Can you work these out from the model? Positions are in its coordinate system, mm. A direction names the side the tool comes from. Round coordinates to 2 decimals unless told otherwise and drop trailing zeros. Order: outer loops, then holes, each group sorted by start corner. A loop starts at its lowest first (then second) coordinate and runs counter-clockwise, first axis right, second up. Notation, with made-up numbers: (39, 9.25) -> (64, 9.25) arc R22 cw to (64, 29.25) -> close; hole circle Ø7 at (7.25, 55). An arc over 180 degrees is marked (long way). Use a Markdown table: item, result. Add a question column.
Q1. For faces 4 (the face through (12, 28, 35)), 5 (the face through (35.651, -4.868, 22.325)), 6 (the face through (-0.66, -29.993, 117.902)), 7 (the face through (-31, 0, 95)), which set-ups out of +Z, -Z, +X, -X, +Y, -Y let a thin tool reach every point of the face, with its end or its side?
Q2. I need wall thicknesses on line 1 along Y through (x, z) = (0, 18); line 2 along Z through (x, y) = (-42.5, -6.5); line 3 along Y through (x, z) = (0, 6.5). Which ranges of each line are inside material? Lowest first, please. Write a range as [from, to].
Q3. If we section it at D-D on z = 57: List the corners of the cut face in (x, y) for me.
Q4. We'd pull the mould along X, two halves only. Please class faces 1 (the face through (-59.94, 2.64, 17.26)), 2 (the face through (31, -18, 76)), 3 (the face through (-48.4, -15.2, 88.1)): +X half, -X half, draft (parallel to the pull), parting line (faces both ways), or undercut.
Q5. If we section it at A-A on z = 88: List the corners of the cut face in (x, y) for me.
Q6. I'm going to push flat-ended pins straight in: pin 1 Ø4 at (x, z) = (-26.5, 100.5) entering from -Y; pin 2 Ø10 at (x, z) = (-46, 26.5) entering from -Y; pin 3 Ø14.5 at (x, y) = (-42, 0) entering from -Z. Where does each tip first touch, or does it pass through?
Q7. If we section it at C-C on x = -45: List the corners of the cut face in (y, z) for me.
Q8. If we section it at B-B on y = -38.5: List the corners of the cut face in (x, z) for me, plus the area to 3 significant figures.
```python
from build123d import *

# Parameters (mm, degrees)
BOSS_EXTRUDE1_DEPTH         = 125
SKETCH1_4_R                 = 12.5
BOSS_EXTRUDE2_DEPTH         = 65
SKETCH1_5_R                 = 60
SKETCH1_5_R_2               = 8
SKETCH1_5_R_3               = 30
BOSS_EXTRUDE3_DEPTH         = 35
BOSS_EXTRUDE4_START         = -49
BOSS_EXTRUDE4_DEPTH         = 35
FILLET1_RADIUS              = 17.5
FILLET1_LENGTH              = 30
F_16_0_16_DIAMETER_HOLE1_D  = 16
FILLET1_OF_MIRROR1_2_RADIUS = 17.5
FILLET1_OF_MIRROR1_2_LENGTH = 30
SKETCH5_R                   = 53.79037733
CUT_EXTRUDE2_DEPTH          = 10


with BuildPart() as part:
    # Sketch1 → Boss-Extrude1 (new body)
    with BuildSketch(Plane.XY):
        with BuildLine():
            Line((30, 0), (20, 0))
            ThreePointArc((20, 0), (0, -20), (-20, 0))
            Line((-20, 0), (-30, 0))
            ThreePointArc((-30, 0), (0, -30), (30, 0))
        make_face()
    extrude(amount=BOSS_EXTRUDE1_DEPTH)

    # Sketch1<4> → Boss-Extrude2 (add)
    with BuildSketch(Plane.XY):
        with BuildLine():
            ThreePointArc((-20, 0), (0, -20), (20, 0))
            Line((20, 0), (30, 0))
            ThreePointArc((30, 0), (0, 30), (-30, 0))
            Line((-30, 0), (-20, 0))
        make_face()
        Circle(SKETCH1_4_R, mode=Mode.SUBTRACT)
    extrude(amount=BOSS_EXTRUDE2_DEPTH)

    # Sketch1<5> → Boss-Extrude3 (add)
    with BuildSketch(Plane.XY):
        Circle(SKETCH1_5_R)
        with Locations((0, 42)):
            Circle(SKETCH1_5_R_2, mode=Mode.SUBTRACT)
        with Locations((-42, 0)):
            Circle(SKETCH1_5_R_2, mode=Mode.SUBTRACT)
        with Locations((0, -42)):
            Circle(SKETCH1_5_R_2, mode=Mode.SUBTRACT)
        with Locations((42, 0)):
            Circle(SKETCH1_5_R_2, mode=Mode.SUBTRACT)
        Circle(SKETCH1_5_R_3, mode=Mode.SUBTRACT)
    extrude(amount=BOSS_EXTRUDE3_DEPTH)

    # Sketch2 → Boss-Extrude4 (add)
    with BuildSketch(Plane.XY.offset(125).offset(BOSS_EXTRUDE4_START)):
        with BuildLine():
            Line((30, 0), (60, 0))
            Line((60, 0), (60, -26.364821455))
            Line((60, -26.364821455), (60, -30))
            Line((60, -30), (0, -30))
            ThreePointArc((0, -30), (21.213203436, -21.213203436), (30, 0))
        make_face()
    boss_extrude4 = extrude(amount=BOSS_EXTRUDE4_DEPTH)

    # Fillet1: full round fillet: the end face becomes a half cylinder, R = half its width
    fillet1_face = Plane((60, -15, 93.5), x_dir=(0, 1, 0), z_dir=(1, 0, 0))  # on the end face: x along it, z out of the body
    fillet1_slab = fillet1_face.offset(-FILLET1_RADIUS / 2) * Box(FILLET1_LENGTH, 2 * FILLET1_RADIUS, FILLET1_RADIUS, mode=Mode.PRIVATE)  # the body's end, R deep
    fillet1_round = Plane((42.5, -15, 93.5), x_dir=(1, 0, 0), z_dir=(0, 1, 0)) * Cylinder(FILLET1_RADIUS, FILLET1_LENGTH, mode=Mode.PRIVATE)  # its axis R under the face
    add(fillet1_slab - fillet1_round, mode=Mode.SUBTRACT)

    # Ø16.0 (16) Diameter Hole1 (through all)
    with Locations(Plane(origin=(42.5, 0, 93.5), x_dir=(1, 0, 0), z_dir=(0, 1, 0))):
        with Locations((0, 0)):
            f_16_0_16_diameter_hole1 = Hole(F_16_0_16_DIAMETER_HOLE1_D / 2)

    # Mirror1: Boss-Extrude4, Ø16.0 (16) Diameter Hole1 across plane
    add(boss_extrude4.mirror(Plane(origin=(0, 0, 0), x_dir=(0, 0, 1), z_dir=(1, 0, 0))))
    add(f_16_0_16_diameter_hole1.mirror(Plane(origin=(0, 0, 0), x_dir=(0, 0, 1), z_dir=(1, 0, 0))), mode=Mode.SUBTRACT)

    # Fillet1 of Mirror1 2: full round fillet: the end face becomes a half cylinder, R = half its width
    fillet1_of_mirror1_2_face = Plane((-60, -15, 93.5), x_dir=(0, 1, 0), z_dir=(-1, 0, 0))  # on the end face: x along it, z out of the body
    fillet1_of_mirror1_2_slab = fillet1_of_mirror1_2_face.offset(-FILLET1_OF_MIRROR1_2_RADIUS / 2) * Box(FILLET1_OF_MIRROR1_2_LENGTH, 2 * FILLET1_OF_MIRROR1_2_RADIUS, FILLET1_OF_MIRROR1_2_RADIUS, mode=Mode.PRIVATE)  # the body's end, R deep
    fillet1_of_mirror1_2_round = Plane((-42.5, -15, 93.5), x_dir=(-1, 0, 0), z_dir=(0, 1, 0)) * Cylinder(FILLET1_OF_MIRROR1_2_RADIUS, FILLET1_OF_MIRROR1_2_LENGTH, mode=Mode.PRIVATE)  # its axis R under the face
    add(fillet1_of_mirror1_2_slab - fillet1_of_mirror1_2_round, mode=Mode.SUBTRACT)

    # Sketch5 → Cut-Extrude2 (cut)
    with BuildSketch(Plane(origin=(0, 0, 0), x_dir=(-1, 0, 0), z_dir=(0, 0, -1))):
        Circle(SKETCH5_R)
    extrude(amount=-CUT_EXTRUDE2_DEPTH, mode=Mode.SUBTRACT)


solid = part.part
```
Answer below:
| question | item | result |
|---|---|---|
| 1 | face 4 | none |
| 1 | face 5 | -Z |
| 1 | face 6 | +Z, -Y |
| 1 | face 7 | +Z, +X, -X, +Y |
| 2 | line 1 | [-60, -50], [-34, -12.5], [12.5, 34], [50, 60] |
| 2 | line 2 | [76, 85.5], [101.5, 111] |
| 2 | line 3 | [-60, -53.79], [53.79, 60] |
| 3 | outline | circle Ø60 at (0, 0); hole circle Ø25 at (0, 0) |
| 4 | face 1 | parting line |
| 4 | face 2 | draft |
| 4 | face 3 | undercut |
| 5 | outline | (-59.11, -30) -> (-48.31, -30) -> (-48.31, 0) -> (-59.11, 0) -> close; (-36.69, -30) -> (36.69, -30) -> (36.69, 0) -> (20, 0) arc R20 cw to (-20, 0) -> (-36.69, 0) -> close; (48.31, -30) -> (59.11, -30) -> (59.11, 0) -> (48.31, 0) -> close |
| 6 | pin 1 | y = -30 |
| 6 | pin 2 | y = -43.81 |
| 6 | pin 3 | z = 76 |
| 7 | outline | (-39.69, 0) -> (-29.47, 0) -> (-29.47, 10) -> (-7.42, 10) -> (-7.42, 35) -> (-39.69, 35) -> close; (-30, 76.18) -> (0, 76.18) -> (0, 85.9) -> (-30, 85.9) -> close; (-30, 101.1) -> (0, 101.1) -> (0, 110.82) -> (-30, 110.82) -> close; (7.42, 10) -> (29.47, 10) -> (29.47, 0) -> (39.69, 0) -> (39.69, 35) -> (7.42, 35) -> close |
| 8 | outline | (-46.02, 0) -> (-37.57, 0) -> (-37.57, 10) -> (-7.19, 10) -> (-7.19, 35) -> (-46.02, 35) -> close; (7.19, 10) -> (37.57, 10) -> (37.57, 0) -> (46.02, 0) -> (46.02, 35) -> (7.19, 35) -> close |
| 8 | area | 2,110 mm² |
